Geometry: final body of the model. Coordinates: model frame, mm. Face numbers are marked on the shaded views. A direction names the side the tool comes from. Coordinates: 2 decimals unless noted, no trailing zeros. Write each loop counter-clockwise with the first axis right and the second up, starting at its lowest first coordinate (ties: lowest second). Pieces come first, ordered by that corner, then holes. Notation, with made-up numbers: (32.25, -38.75) -> (87.25, -38.75) arc R25 cw to (87.25, -17.75) -> close; hole circle Ø6 at (40.5, -2). An arc over 180 degrees is marked (long way). One line per item, written item: value. Start each with the question number.
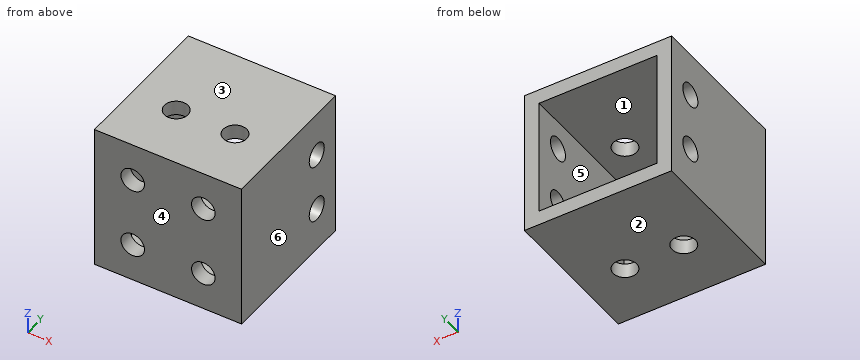
from build123d import *

# Parameters (mm, degrees)
SKETCH1_W               = 50
SKETCH1_H               = 50
BOSS_EXTRUDE1_DEPTH     = 50
SKETCH2_W               = 40
SKETCH2_H               = 40
CUT_EXTRUDE1_DEPTH      = 45
SKETCH3_R               = 4
CUT_EXTRUDE2_DEPTH      = 45
CUT_EXTRUDE3_DEPTH      = 87.602540378
CUT_EXTRUDE3_DEPTH_BACK = 87.602540378
SKETCH4_R               = 4
CUT_EXTRUDE4_DEPTH      = 87.602540378
CUT_EXTRUDE4_DEPTH_BACK = 87.602540378
SKETCH5_R               = 4


with BuildPart() as part:
    # Sketch1 → Boss-Extrude1 (new body)
    with BuildSketch(Plane(origin=(0, 0, 0), x_dir=(1, 0, 0), z_dir=(0, 1, 0))):
        with Locations((25, 25)):
            Rectangle(SKETCH1_W, SKETCH1_H)
    extrude(amount=BOSS_EXTRUDE1_DEPTH)

    # Sketch2 → Cut-Extrude1 (cut)
    with BuildSketch(Plane(origin=(0, 50, 0), x_dir=(1, 0, 0), z_dir=(0, 1, 0))):
        with Locations((25, 25)):
            Rectangle(SKETCH2_W, SKETCH2_H)
    extrude(amount=-CUT_EXTRUDE1_DEPTH, mode=Mode.SUBTRACT)

    # Sketch3 → Cut-Extrude2 (cut)
    with BuildSketch(Plane(origin=(0, 5, 0), x_dir=(1, 0, 0), z_dir=(0, 1, 0))):
        with Locations(Location((13, 37, 0), (0, 0, 270))):
            Circle(SKETCH3_R)
        with Locations(Location((37, 37, 0), (0, 0, 270))):
            Circle(SKETCH3_R)
        with Locations(Location((13, 13, 0), (0, 0, 270))):
            Circle(SKETCH3_R)
        with Locations(Location((37, 13, 0), (0, 0, 270))):
            Circle(SKETCH3_R)
    extrude(amount=-CUT_EXTRUDE2_DEPTH, mode=Mode.SUBTRACT)

    # Sketch4 → Cut-Extrude3 (cut, two sides: drawn at the far end of the back side and taken through both)
    with BuildSketch(Plane.XY.offset(-CUT_EXTRUDE3_DEPTH_BACK)):
        with Locations((15, 20)):
            Circle(SKETCH4_R)
        with Locations((35, 20)):
            Circle(SKETCH4_R)
    extrude(amount=CUT_EXTRUDE3_DEPTH + CUT_EXTRUDE3_DEPTH_BACK, mode=Mode.SUBTRACT)

    # Sketch5 → Cut-Extrude4 (cut, two sides: drawn at the far end of the back side and taken through both)
    with BuildSketch(Plane(origin=(50, 0, 0), x_dir=(0, 0, -1), z_dir=(1, 0, 0)).offset(-CUT_EXTRUDE4_DEPTH_BACK)):
        with Locations((15, 40)):
            Circle(SKETCH5_R)
        with Locations((35, 40)):
            Circle(SKETCH5_R)
    extrude(amount=CUT_EXTRUDE4_DEPTH + CUT_EXTRUDE4_DEPTH_BACK, mode=Mode.SUBTRACT)


solid = part.part
Q1. First-contact query: P1, Ø9, axis at x = 37, z = -13, coming from the +Y side. Flat tip, straight axial feed; report the tip coordinate or a pass-through.
Q2. Line query: L1, parallel to X at y = 3.55, z = -13; L2, parallel to Z at x = 3.25, y = 40; L3, parallel to X at y = 24.5, z = -12. Output: solid intervals per line, ascending. Write a range as from..to.
Q3. Cut plane B-B on z = -36. Output: boundary loops of the cut face in (x, y), and give its area (3 significant figures).
Q4. Draft query along Z for the marked faces 1, 2, 3 and 4. Return one class per face: pulls with the +Z half, pulls with the -Z half, needs draft (parallel to the pull), parting line crosses it, or undercut.
Q5. Cut plane D-D on y = 46. Output: boundary loops of the cut face in (x, z).
Q6. Cut plane A-A on x = 12. Output: boundary loops of the cut face in (y, z), and give its area (3 significant figures).
Q7. Access query for the marked faces 5 and 6. Directions: +Z, -Z, +X, -X, +Y, -Y. A direction counts if a zero-diameter tool reaches every point of the face in a straight line with its end or side. Return the directions, or none.
Q8. Cut plane C-C on y = 20. Output: boundary loops of the cut face in (x, z), and give its area (3 significant figures).
Solution:
1. P1: y = 5
2. L1: 0..9, 17..33, 41..50
2. L2: -50..-39, -31..-19, -11..0
2. L3: 0..5, 45..50
3. outline: (0, 0) -> (9.13, 0) -> (9.13, 5) -> (5, 5) -> (5, 36.13) -> (0, 36.13) -> close; (0, 43.87) -> (5, 43.87) -> (5, 50) -> (0, 50) -> close; (16.87, 0) -> (33.13, 0) -> (33.13, 5) -> (16.87, 5) -> close; (40.87, 0) -> (50, 0) -> (50, 36.13) -> (45, 36.13) -> (45, 5) -> (40.87, 5) -> close; (45, 43.87) -> (50, 43.87) -> (50, 50) -> (45, 50) -> close
3. area: 545 mm²
4. face 1: undercut
4. face 2: pulls with the -Z half
4. face 3: pulls with the +Z half
4. face 4: needs draft
5. outline: (0, -50) -> (50, -50) -> (50, 0) -> (0, 0) -> close; hole (5, -45) -> (45, -45) -> (45, -5) -> (5, -5) -> close
6. outline: (0, -50) -> (17.35, -50) -> (17.35, -45) -> (5, -45) -> (5, -40.87) -> (0, -40.87) -> close; (0, -33.13) -> (5, -33.13) -> (5, -16.87) -> (0, -16.87) -> close; (0, -9.13) -> (5, -9.13) -> (5, -5) -> (17.35, -5) -> (17.35, 0) -> (0, 0) -> close; (22.65, -50) -> (50, -50) -> (50, -45) -> (22.65, -45) -> close; (22.65, -5) -> (50, -5) -> (50, 0) -> (22.65, 0) -> close
6. area: 570 mm²
7. face 5: +Y
7. face 6: +Z, -Z, +X, +Y, -Y
8. outline: (0, -50) -> (11, -50) -> (11, -45) -> (5, -45) -> (5, -5) -> (11, -5) -> (11, 0) -> (0, 0) -> close; (19, -50) -> (31, -50) -> (31, -45) -> (19, -45) -> close; (19, -5) -> (31, -5) -> (31, 0) -> (19, 0) -> close; (39, -50) -> (50, -50) -> (50, 0) -> (39, 0) -> (39, -5) -> (45, -5) -> (45, -45) -> (39, -45) -> close
8. area: 740 mm²
